from build123d import *

# Parameters (mm, degrees)
SKETCH1_R           = 6.35
SKETCH1_R_2         = 1.5875
SKETCH1_R_3         = 3.175
BOSS_EXTRUDE1_DEPTH = 2.54


with BuildPart() as part:
    # Sketch1 → Boss-Extrude1 (new body)
    # profile 1 of 3: a face of its own
    with BuildSketch(Plane.XY):
        Circle(SKETCH1_R)
        Circle(SKETCH1_R_2, mode=Mode.SUBTRACT)
    # profile 2 of 3: a face of its own
    with BuildSketch(Plane.XY):
        with BuildLine():
            Line((98.5266, 6.35), (0, 6.35))
            ThreePointArc((0, 6.35), (4.490128061, 4.490128061), (6.35, 0))
            ThreePointArc((6.35, 0), (4.490128061, -4.490128061), (0, -6.35))
            Line((0, -6.35), (98.5266, -6.35))
            ThreePointArc((98.5266, -6.35), (92.1766, 0), (98.5266, 6.35))
        make_face()
        with Locations((19.05, 0)):
            Circle(SKETCH1_R_3, mode=Mode.SUBTRACT)
        with Locations((79.4766, 0)):
            Circle(SKETCH1_R_3, mode=Mode.SUBTRACT)
    # profile 3 of 3: a face of its own
    with BuildSketch(Plane.XY):
        with Locations((98.5266, 0)):
            Circle(SKETCH1_R)
        with Locations((98.5266, 0)):
            Circle(SKETCH1_R_2, mode=Mode.SUBTRACT)
    extrude(amount=BOSS_EXTRUDE1_DEPTH)


solid = part.part
Build history of the part. All positions in model axes, mm. Round coordinates to 2 decimals unless told otherwise and drop trailing zeros. Write each loop counter-clockwise with the first axis right and the second up, starting at its lowest first coordinate (ties: lowest second). Pieces come first, ordered by that corner, then holes. Notation, with made-up numbers: (74, 43) -> (121, 43) arc R23 cw to (121, 57) -> close; hole circle Ø9 at (72.5, 20.5). An arc over 180 degrees is marked (long way). Write item = value, one per line.
(1) Band-saw the part on A-A (y = 0). State how many separate pieces and enclosed holes the cut face has, then the cut area to 3 significant figures.
Answer:
separate_pieces = 5
enclosed_holes = 0
area = 234 mm2
(2) Band-saw the part on B-B (x = 19.05). Give the cut face in (y, z) (3 decimals).
Answer:
outline = (-6.35, 0) -> (-3.175, 0) -> (-3.175, 2.54) -> (-6.35, 2.54) -> close; (3.175, 0) -> (6.35, 0) -> (6.35, 2.54) -> (3.175, 2.54) -> close
(3) Probe L1, parallel to X at y = -1.25, z = 2.3; L2, parallel to Y at x = 19.05, z = 1.9 (3 decimals); L3, parallel to X at y = -1, z = 0.85. List the from-to ranges inside material, lowest first.
Answer:
L1 = -6.23 to -0.98, 0.98 to 16.13, 21.97 to 76.56, 82.4 to 97.55, 99.51 to 104.75
L2 = -6.35 to -3.175, 3.175 to 6.35
L3 = -6.27 to -1.23, 1.23 to 16.04, 22.06 to 76.46, 82.49 to 97.29, 99.76 to 104.8
(4) Two-plate mould, pull along Y, no slides. Class faces 1 (the face through (48, 0, 0)), 2 (the face through (49, -6.35, 1)), 3 (the face through (96.94, 0.07, 1.25)): pulls with the +Y half, pulls with the -Y half, needs draft (parallel to the pull), parting line crosses it, or undercut.
Answer:
face_1 = needs draft
face_2 = pulls with the -Y half
face_3 = undercut
